from build123d import *


with BuildPart() as part:
    # Sketch1 → Revolve1 (revolve)
    with BuildSketch(Plane.XY):
        with BuildLine():
            Line((13.5, 25), (-13.5, 25))
            ThreePointArc((-13.5, 25), (-14.914213562, 25.585786438), (-15.5, 27))
            Line((-15.5, 27), (-15.5, 37))
            Line((-15.5, 37), (-8.94427191, 37))
            ThreePointArc((-8.94427191, 37), (0, 33), (8.94427191, 37))
            Line((8.94427191, 37), (15.5, 37))
            Line((15.5, 37), (15.5, 27))
            ThreePointArc((15.5, 27), (14.914213562, 25.585786438), (13.5, 25))
        make_face()
    revolve(axis=Axis((-15.5, 0, 0), (1, 0, 0)))


solid = part.part
Verification items for the finished model (mm, model axes). Round coordinates to 2 decimals unless told otherwise and drop trailing zeros. Order: outer loops, then holes, each group sorted by start corner. A loop starts at its lowest first (then second) coordinate and runs counter-clockwise, first axis right, second up. Notation, with made-up numbers: (51, -38) -> (69, -38) arc R24 ccw to (69, -25) -> close; hole circle Ø9 at (63, 84.5). An arc over 180 degrees is marked (long way). Put each result on its own line as item: value.
1) Section check A-A (y = 0). Record the cut outline in (x, z).
Final values:
outline: (-15.5, -37) -> (-8.94, -37) arc R12 cw to (8.94, -37) -> (15.5, -37) -> (15.5, -27) arc R2 ccw to (13.5, -25) -> (-13.5, -25) arc R2 ccw to (-15.5, -27) -> close; (-15.5, 27) arc R2 ccw to (-13.5, 25) -> (13.5, 25) arc R2 ccw to (15.5, 27) -> (15.5, 37) -> (8.94, 37) arc R12 cw to (-8.94, 37) -> (-15.5, 37) -> close
2) Depth check by flat-ended pin: pin 1 (1.5 mm diameter, centred on x = 2, y = 22, fed in from -Z); pin 2 (3 mm diameter, centred on x = 9.5, y = -17.5, fed in from -Z); pin 3 (3 mm diameter, centred on x = 9, z = 12.5, fed in from -Y). Enter the tip coordinate at first touch or a pass-through.
Final values:
pin 1: stops at z = -25.49
pin 2: stops at z = -33.36
pin 3: stops at y = -35.33
3) Section check D-D (x = 0). Record the cut outline in (y, z).
Final values:
outline: circle Ø66 at (0, 0); hole circle Ø50 at (0, 0)
4) Mould release check, pull along Y, two halves, no side actions. Record for faces 1 (the cylindrical face through (-12.18, -8.02, -36.12)), 2 (the flat face through (-15.5, -3, -27)), 3 (the cylindrical face through (-0.189, 23.846, 7.509)): +Y half, -Y half, draft (parallel to the pull), parting line (faces both ways), or undercut.
Final values:
face 1: parting line
face 2: draft
face 3: undercut
5) Material ranges on line 1 (Y direction, x = -6, z = -4); line 2 (Z direction, x = 4.5, y = 0); line 3 (Z direction, x = 0, y = -7.5), recorded low to high.
Final values:
line 1: y = -34.38 to -24.68, 24.68 to 34.38
line 2: z = -33.88 to -25, 25 to 33.88
line 3: z = -32.14 to -23.85, 23.85 to 32.14
6) Section check C-C (x = 12.5). Record the cut outline in (y, z).
Final values:
outline: circle Ø74 at (0, 0); hole circle Ø50 at (0, 0)
